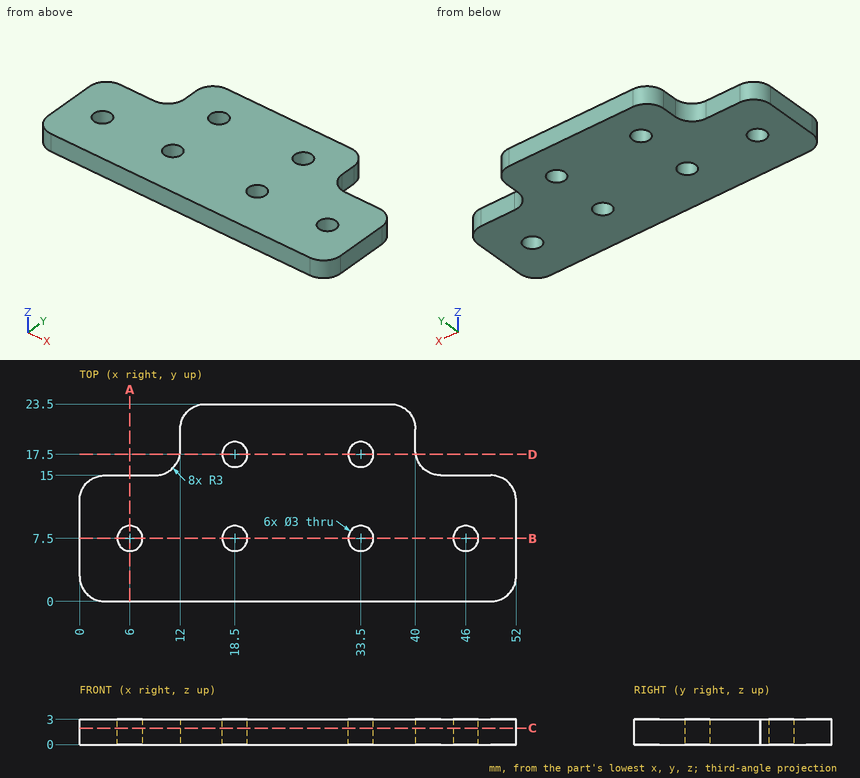
Geometry check sheet. Reference: drawing and pictorial views, mm from the part's lowest x, y, z. Give positions to 0.01 mm unless a question says otherwise; leave off trailing zeros. Order: outer loops, then holes, each group sorted by start corner. A loop starts at its lowest first (then second) coordinate and runs counter-clockwise, first axis right, second up. Notation, with made-up numbers: M -0.75,51 L 36.25,51 A16 ccw 36.25,56 Z; hole C 19,22 d6. An arc over 180 degrees is marked long. Answer in a Markdown table with one row per item. Add a question column.
Q1. Gauge pin test, flat ends, axial feed: pin 1 Ø1.5 at (x, z) = (6.5, 1.5) entering from +Y; pin 2 Ø1.2 at (y, z) = (20, 1.5) entering from +X; pin 3 Ø4 at (x, y) = (46, 7.5) entering from +Z; pin 4 Ø0.8 at (y, z) = (19, 1.5) entering from -X. Record the tip position at first contact, or that the pin passes through.
Q2. Sectioned sample at D-D, the plane y = 17.5. Record the boundary of the cut face in (x, z).
Q3. Sectioned sample at B-B, the plane y = 7.5. Record the boundary of the cut face in (x, z).
Q4. Sectioned sample at A-A, the plane x = 6. Record the boundary of the cut face in (y, z), and give its area (3 significant figures).
Q5. Sectioned sample at C-C, the plane z = 1.95. Record the boundary of the cut face in (x, y).
Q6. Thickness scan on L1, parallel to Y at x = 18.5, z = 1.6; L2, parallel to Y at x = 6, z = 0.85; L3, parallel to X at y = 8, z = 2.65. Record the ranges inside material, lowest first.
Verdict:
| question | item | result |
|---|---|---|
| 1 | pin 1 | y = 15 |
| 1 | pin 2 | x = 40 |
| 1 | pin 3 | z = 3 |
| 1 | pin 4 | x = 12 |
| 2 | outline | M 11.96,0 L 17,0 L 17,3 L 11.96,3 Z; M 20,0 L 32,0 L 32,3 L 20,3 Z; M 35,0 L 40.04,0 L 40.04,3 L 35,3 Z |
| 3 | outline | M 0,0 L 4.5,0 L 4.5,3 L 0,3 Z; M 7.5,0 L 17,0 L 17,3 L 7.5,3 Z; M 20,0 L 32,0 L 32,3 L 20,3 Z; M 35,0 L 44.5,0 L 44.5,3 L 35,3 Z; M 47.5,0 L 52,0 L 52,3 L 47.5,3 Z |
| 4 | outline | M 0,0 L 6,0 L 6,3 L 0,3 Z; M 9,0 L 15,0 L 15,3 L 9,3 Z |
| 4 | area | 36.0 mm² |
| 5 | outline | M 0,3 A3 ccw 3,0 L 49,0 A3 ccw 52,3 L 52,12 A3 ccw 49,15 L 43,15 A3 cw 40,18 L 40,20.5 A3 ccw 37,23.5 L 15,23.5 A3 ccw 12,20.5 L 12,18 A3 cw 9,15 L 3,15 A3 ccw 0,12 Z; hole C 6,7.5 d3; hole C 18.5,7.5 d3; hole C 18.5,17.5 d3; hole C 33.5,7.5 d3; hole C 33.5,17.5 d3; hole C 46,7.5 d3 |
| 6 | L1 | 0 to 6, 9 to 16, 19 to 23.5 |
| 6 | L2 | 0 to 6, 9 to 15 |
| 6 | L3 | 0 to 4.59, 7.41 to 17.09, 19.91 to 32.09, 34.91 to 44.59, 47.41 to 52 |
